Part model, mm, in its own coordinate system. Coordinates: 2 decimals unless noted, no trailing zeros. Loops run counter-clockwise (first coordinate to the right, second up) from the corner with the lowest first, then second, coordinate; pieces in that order, holes last. Notation, with made-up numbers: M 75,67 L 129,67 A23 ccw 129,94 Z; hole C 58.5,59 d8. An arc over 180 degrees is marked long. Answer as a JSON object with one key per item and string values. Group by question number.
1. Drop flat-ended pins along their axis: pin 1 Ø4.5 at (x, y) = (-68.98, -3.48) entering from +Z; pin 2 Ø0.9 at (y, z) = (-208.5, 2) entering from -X; pin 3 Ø1 at (y, z) = (-66.5, 1) entering from -X. Give the stop position or say it passes through.
2. Saw through at C-C on x = 54. Write the cut outline in (y, z), then the cut area to 3 significant figures.
3. Saw through at A-A on x = 204. Write the cut outline in (y, z), then the cut area to 3 significant figures.
4. Drill centre lines: L1, parallel to Y at x = -149.5, z = 0.35; L2, parallel to X at y = -180, z = 1.3; L3, parallel to X at y = 53, z = 2.7. Where is each one in solid material? Low to high.
5. Saw through at B-B on z = 1.5. Count the separate pieces of the cut face and the enclosed holes in it, then the cut area to 3 significant figures.
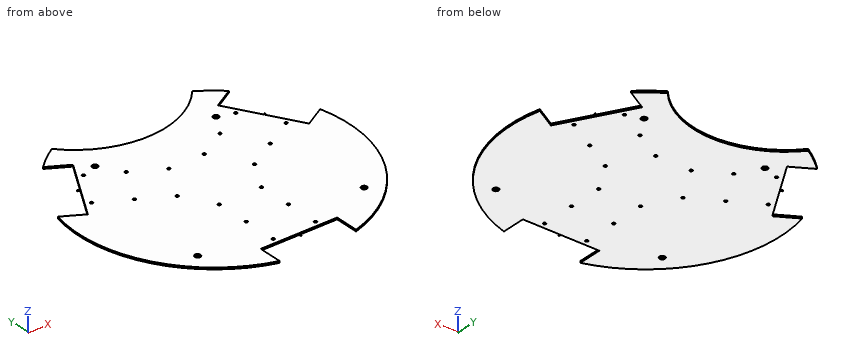
Autodesk Fusion 360 part; units mm, degrees
sketch "Esboço1" plane through (0, 0, 0) normal (0, 0, 1) x (1, 0, 0)
  circle A0 centre (0, 0) radius 240
  circle A1 centre (148, -148) radius 5
  line L0 (-125, 204.878) -> (125, 204.878)
  circle A2 centre (0, 311.043) radius 164
  circle A3 centre (107.5, 130.5) radius 5
  line L1 (-40, 115) -> (40, 115)
  line L2 (-40, 115) -> (-40, 151.9958)
  line L3 (40, 115) -> (40, 151.9958)
  line L4 (0, 1.75) -> (0, 22.5)
  circle A4 centre (-148, -148) radius 5
  circle A5 centre (-107.5, 130.5) radius 5
  line L5 (-68, -188) -> (68, -188)
  line L6 (68, -188) -> (68, -240)
  line L7 (68, -240) -> (-68, -240)
  line L8 (-68, -240) -> (-68, -188)
  line L9 (0, -188) -> (0, -178)
  line L10 (-37.5, -178) -> (37.5, -178)
  circle A6 centre (-37.5, -178) radius 2.5
  circle A7 centre (37.5, -178) radius 2.5
  circle A8 centre (37.5, -118) radius 2.5
  circle A9 centre (37.5, -58) radius 2.5
  circle A10 centre (-37.5, -118) radius 2.5
  circle A11 centre (-37.5, -58) radius 2.5
  circle A12 centre (135.4025, 121.476) radius 2.5
  line L11 (241.8461, 61.1103) -> (196.8128, 35.1103)
  line L12 (196.8128, 35.1103) -> (128.8128, 152.8897)
  line L13 (128.8128, 152.8897) -> (173.8461, 178.8897)
  circle A13 centre (83.441, 91.476) radius 2.5
  circle A14 centre (172.9025, 56.524) radius 2.5
  circle A15 centre (120.941, 26.524) radius 2.5
  circle A16 centre (68.9795, -3.476) radius 2.5
  circle A17 centre (31.4795, 61.476) radius 2.5
  circle A18 centre (-172.9025, 56.524) radius 2.5
  line L14 (-173.8461, 178.8897) -> (-128.8128, 152.8897)
  line L15 (-128.8128, 152.8897) -> (-196.8128, 35.1103)
  line L16 (-196.8128, 35.1103) -> (-241.8461, 61.1103)
  circle A19 centre (-120.941, 26.524) radius 2.5
  circle A20 centre (-135.4025, 121.476) radius 2.5
  circle A21 centre (-83.441, 91.476) radius 2.5
  circle A22 centre (-31.4795, 61.476) radius 2.5
  circle A23 centre (-68.9795, -3.476) radius 2.5
  point P0 (0, 115)
  point P1 (0, -240)
  point P2 (-68, -230.1652)
  dimension "d1" = 480
  dimension "d13" = 10
  dimension "d14" = 148
  dimension "d15" = 148
  dimension "d16" = 250
  dimension "d17" = 328
  dimension "d18" = 10
  dimension "d19" = 130.5
  dimension "d20" = 107.5
  dimension "d21" = 115
  dimension "d22" = 80
  dimension "d25" = 136
  dimension "d26" = 52
  dimension "d27" = 10
  dimension "d28" = 75
  dimension "d29" = 5
  dimension "d30" = 5
  dimension "d33" = 1
  dimension "d34" = 60
  dimension "d36" = 360
extrude "Extrusão1" add sketch "Esboço1" along normal blind 3 contours A0 A2 L1 L2 L3 L5 L6 L8 L11 L12 L13 L14 L15 L16 | A2 L1 L2 L3
sketch "Esboço2" plane through (162.8128, 94, 0) normal (0.866, 0.5, 0) x (-0.5, 0.866, 0)
  line L0 (-68, 0) -> (68, 0)
  line L1 (68, 0) -> (68, 3)
  line L2 (68, 3) -> (-68, 3)
  line L3 (-68, 3) -> (-68, 0)
  line L4 (68, 0) -> (-68, 0)
  line L5 (-68, 0) -> (-68, 3)
  line L6 (-68, 3) -> (68, 3)
  line L7 (68, 3) -> (68, 0)
  line L8 (0, 0) -> (0, 3) construction
  line L9 (-68, 1.5) -> (68, 1.5) construction
  circle A0 centre (0, 1.5) radius 0.75
  dimension "d38" = 1.5
sketch "Esboço3" plane through (0, -188, 0) normal (0, -1, 0) x (1, 0, 0)
  line L0 (-68, 0) -> (68, 0)
  line L1 (68, 0) -> (68, 3)
  line L2 (68, 3) -> (-68, 3)
  line L3 (-68, 3) -> (-68, 0)
  line L4 (68, 0) -> (-68, 0)
  line L5 (-68, 0) -> (-68, 3)
  line L6 (-68, 3) -> (68, 3)
  line L7 (68, 3) -> (68, 0)
  line L8 (0, 0) -> (0, 3) construction
  line L9 (-68, 1.5) -> (68, 1.5) construction
  circle A0 centre (0, 1.5) radius 0.75
  dimension "d39" = 1.5
sketch "Esboço4" plane through (-162.8128, 94, 0) normal (-0.866, 0.5, 0) x (-0.5, -0.866, 0)
  line L0 (-68, 0) -> (68, 0)
  line L1 (68, 0) -> (68, 3)
  line L2 (68, 3) -> (-68, 3)
  line L3 (-68, 3) -> (-68, 0)
  line L4 (68, 0) -> (-68, 0)
  line L5 (-68, 0) -> (-68, 3)
  line L6 (-68, 3) -> (68, 3)
  line L7 (68, 3) -> (68, 0)
  line L8 (0, 0) -> (0, 3) construction
  line L9 (68, 1.5) -> (-68, 1.5) construction
  circle A0 centre (0, 1.5) radius 0.75
  dimension "d40" = 1.5
extrude "Extrusão2" add sketch "Esboço4" along normal blind 5 contours A0
extrude "Extrusão3" add sketch "Esboço2" along normal blind 5 contours A0
extrude "Extrusão4" add sketch "Esboço3" along normal blind 5 contours A0
equation "d17 = ( 164 * 2 ) * 1 mm"
Outcome:
{
 "1": {"pin 1": "passes through", "pin 2": "stops at x = -119.65", "pin 3": "stops at x = -230.75"},
 "2": {"outline": "M -188,0 L 156.19,0 L 156.19,3 L -188,3 Z", "area": "1,030 mm²"},
 "3": {"outline": "M -126.43,0 L 39.26,0 L 39.26,3 L -126.43,3 Z", "area": "497 mm²"},
 "4": {"L1": "y = -187.75 to -152.77, -143.23 to 117.06, 164.83 to 187.75", "L2": "x = -158.75 to -39, -36 to 36, 39 to 158.75", "L3": "x = -234.07 to -227.8, -186.48 to 186.48, 227.8 to 234.07"},
 "5": {"separate pieces": "1", "enclosed holes": "22", "area": "144,000 mm²"}
}
